Verification items for this drawing (mm, ordinates from the low corner). A direction names the side the tool comes from. Coordinates: 2 decimals unless noted, no trailing zeros. Write each loop counter-clockwise with the first axis right and the second up, starting at its lowest first coordinate (ties: lowest second). Pieces come first, ordered by that corner, then holes. Notation, with made-up numbers: M 64,83 L 100,83 A38 ccw 100,121 Z; hole C 73,-17.75 d3. An arc over 180 degrees is marked long. Put each result on its own line as item: value. Start each with the question number.
1) Gauge pin test, flat ends, axial feed: pin 1 (1.5 mm diameter, centred on y = 22.5, z = 2, fed in from +X); pin 2 (8 mm diameter, centred on x = 10, y = 10, fed in from -Z). Record the tip position at first contact, or that the pin passes through.
2) Cross-section at D-D on y = 7. Record the cut outline in (x, z), plus the area to 3 significant figures.
3) Set-up check for the marked faces 1, 2 and 3: record each of +Z, -Z, +X, -X, +Y, -Y from which the full face is reachable in a straight line by a thin tool's end or side.
4) Scan lines: line 1 along Y through (x, z) = (10, 1.65) (1 decimal); line 2 along Y through (x, z) = (11.5, 0.7); line 3 along Y through (x, z) = (8, 2.8) (1 decimal). Record each from-to range of solid material in increasing order.
5) Mould release check, pull along Y, two halves, no side actions. Record for the marked faces 4, 5 and 6: released by +Y, released by -Y, zero draft, split by the parting line, or undercut.
6) Cross-section at B-B on y = 10. Record the cut outline in (x, z).
7) Cross-section at C-C on z = 2.85. Record the cut outline in (x, y).
8) Cross-section at A-A on x = 8.25. Record the cut outline in (y, z) (1 decimal).
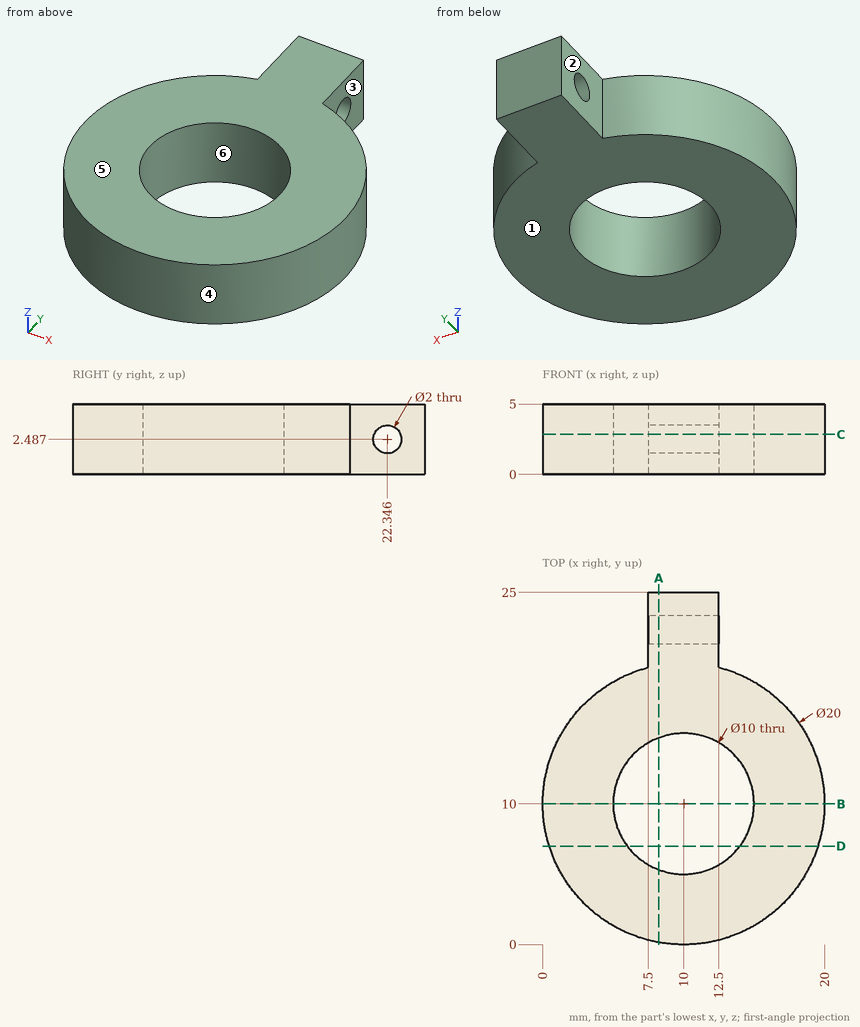
Answer key:
1. pin 1: stops at x = 12.5
1. pin 2: passes through
2. outline: M 0.46,0 L 6,0 L 6,5 L 0.46,5 Z; M 14,0 L 19.54,0 L 19.54,5 L 14,5 Z
2. area: 55.4 mm²
3. face 1: -Z, +X, -X, +Y, -Y
3. face 2: +Z, -Z, -X, +Y
3. face 3: +Z, -Z, +X, +Y
4. line 1: y = 0 to 5, 15 to 21.8, 22.9 to 25
4. line 2: y = 0.11 to 5.23, 14.77 to 25
4. line 3: y = 0.2 to 5.4, 14.6 to 21.4, 23.3 to 25
5. face 4: split by the parting line
5. face 5: zero draft
5. face 6: undercut
6. outline: M 0,0 L 5,0 L 5,5 L 0,5 Z; M 15,0 L 20,0 L 20,5 L 15,5 Z
7. outline: M 7.5,19.68 A10 ccw long 12.5,19.68 L 12.5,21.41 L 7.5,21.41 Z; M 7.5,23.28 L 12.5,23.28 L 12.5,25 L 7.5,25 Z; hole C 10,10 d10
8. outline: M 0.2,0 L 5.3,0 L 5.3,5 L 0.2,5 Z; M 14.7,0 L 25,0 L 25,5 L 14.7,5 Z; hole C 22.3,2.5 d2
